Source: CAD feature listing. Evaluate the final solid. Frame: model axes, mm. Face numbers are marked on the shaded views. A direction names the side the tool comes from. Coordinates: 2 decimals unless noted, no trailing zeros. Order: outer loops, then holes, each group sorted by start corner. A loop starts at its lowest first (then second) coordinate and runs counter-clockwise, first axis right, second up. Notation, with made-up numbers: (63, -34) -> (115, -34) arc R22 cw to (115, -3) -> close; hole circle Ø5 at (79.5, -1). An arc over 180 degrees is marked (long way). Write item = value, one per line. Start each with the question number.
Item 1: Section query D-D (x = 23). Output: boundary loops of the cut face in (y, z), then the cut area to 3 significant figures.
Item 2: Set-up query: the marked faces 1 and 2. Return all of +Z, -Z, +X, -X, +Y, -Y with unobstructed straight access to the full face (end or side cutting, diameter ignored); none if empty.
Item 3: Section query C-C (y = 20). Output: boundary loops of the cut face in (x, z).
Item 4: Contact query for flat-ended pins moving along their axis: pin 1 (3 mm diameter, centred on y = 41.5, z = 18, fed in from -X); pin 2 (1.3 mm diameter, centred on y = 34.5, z = 10, fed in from +X); pin 3 (4 mm diameter, centred on y = 46.5, z = 17, fed in from +X); pin 4 (2 mm diameter, centred on x = -2.5, y = 30, fed in from +Z). Output: stop coordinate, or through.
Item 5: Ray query, line 1 along Z through (x, y) = (6.5, 31); line 2 along Y through (x, z) = (9, -0.5); line 3 along Y through (x, z) = (17, -0.5). Return the intervals inside material, ascending. Write a range as [from, to].
Item 6: Section query A-A (z = 18.5). Output: boundary loops of the cut face in (x, y), then the cut area to 3 significant figures.
Item 7: Section query B-B (x = 34). Output: boundary loops of the cut face in (y, z), then the cut area to 3 significant figures.
```python
from build123d import *

# Parameters (mm, degrees)
F0_W         = 25
F0_H         = 33
F1_DEPTH     = 25
F3_DEPTH     = 10
F5_DEPTH     = 81.7
F7_DEPTH     = 10
F9_DEPTH     = 92
F10_W        = 13
F10_H        = 13
F11_DEPTH    = 40
F12_R        = 1.9
F13_DEPTH    = 7
F15_DEPTH    = 2.5
F16_W        = 78.4268817365
F16_H        = 25
F17_DEPTH    = 2.5
F19_DEPTH    = 336
F21_DEPTH    = 25
F23_W        = 90.9570492804
F23_H        = 10.3441323154
F24_DEPTH    = 48.1
F26_DEPTH    = 199
F27_W        = 183.3121031523
F27_H        = 83.9067064226
F28_DEPTH    = 179
F29_T1_DEPTH = 32.3950995948
F29_T3_DEPTH = 10.395099863
F31_DEPTH    = 25
F32_R        = 1.9
F33_DEPTH    = 25


# Not quite as in the source:
# - a fillet or chamfer that OpenCascade refuses, or shapes differently, is made with other operations: its cross-section is extruded or revolved along the edge and cut away or added


with BuildPart() as f1:
    # F0 (on Top) → F1 (new body)
    with BuildSketch(Plane.XY):
        with Locations((12.5, 16.5)):
            Rectangle(F0_W, F0_H)
        Polygon((-25, 25.3567329635), (0, 0), (0, 33), align=None)
        with Locations((37.5, 16.5)):
            Rectangle(F0_W, F0_H)
        Polygon((25, 40.6432670365), (0, 33), (25, 33), align=None)
        Polygon((0, 101.4598330308), (0, 33), (25, 40.6432670365), (25, 101.4598330308), (25, 137), (0, 137), align=None)
        Polygon((25, 40.6432670365), (25, 33), (50, 33), (50, 48.2865340729), align=None)
        Polygon((-25, 131.6860859582), (0, 101.4598330308), (0, 137), align=None)
        Polygon((25, 137), (25, 101.4598330308), (50, 131.6860859582), (50, 147.6278280835), (25, 142.3139140418), align=None)
        Polygon((25, 142.3139140418), (0, 137), (25, 137), align=None)
        Polygon((0, 177), (0, 137), (25, 142.3139140418), (25, 177), align=None)
    extrude(amount=F1_DEPTH)

    # F2 (on face) → F3 (join)
    with BuildSketch(Plane(origin=(0, 0, 0), x_dir=(1, 0, 0), z_dir=(0, 0, -1))):
        Polygon((50, -131.6860859582), (25, -101.4598330308), (0, -101.4598330308), (-25, -131.6860859582), (50, -147.6278280835), align=None)
    extrude(amount=F3_DEPTH)

    # F4 (on face) → F5 (cut, symmetric)
    with BuildSketch(Plane.YZ.offset(25)):
        Polygon((101.4598330308, -21.1370438337), (147.6278330308, -10), (101.4598330308, 0), align=None)
    extrude(amount=F5_DEPTH, both=True, mode=Mode.SUBTRACT)

    # F6 (on face) → F7 (join)
    with BuildSketch(Plane(origin=(0, 0, 0), x_dir=(1, 0, 0), z_dir=(0, 0, -1))):
        Polygon((50, -48.2865340729), (50, 0), (0, 0), (-25, -25.3567329635), align=None)
    extrude(amount=F7_DEPTH)

    # F8 (on face) → F9 (cut)
    with BuildSketch(Plane.YZ.offset(50)):
        Polygon((48.2865340729, -10), (0, 0), (0, -39.534393698), (48.2865340729, -39.534393698), align=None)
    extrude(amount=-F9_DEPTH, mode=Mode.SUBTRACT)

    # F10 (on face) → F11 (cut)
    with BuildSketch(Plane(origin=(0, 177, 0), x_dir=(-1, 0, 0), z_dir=(0, 1, 0))):
        with Locations((-12.5, 12.5)):
            Rectangle(F10_W, F10_H)
    extrude(amount=-F11_DEPTH, mode=Mode.SUBTRACT)

    # F12 (on face) → F13 (cut)
    with BuildSketch(Plane(origin=(-27.8614600507, 131.0778638485, 0), x_dir=(-0.9781476007, -0.2079116908, 0), z_dir=(-0.2079116908, 0.9781476007, 0))):
        with Locations((-18.6253867704, 12.5)):
            Circle(F12_R)
        with BuildLine():
            ThreePointArc((-72.2009313853, 12.5), (-70.3009313853, 10.6), (-68.4009313853, 12.5))
            ThreePointArc((-68.4009313853, 12.5), (-70.3009313853, 14.4), (-72.2009313853, 12.5))
        make_face()
    extrude(amount=-F13_DEPTH, mode=Mode.SUBTRACT)

    # F15 (add): a face of the model
    f15_faces = [f1.faces().sort_by_distance(p)[0] for p in [
        (12.5, 36.8216335182, -0.8588233683),
    ]]
    extrude(f15_faces, amount=F15_DEPTH)

    # F16 (on face) → F17 (join)
    with BuildSketch(Plane(origin=(-9.9576121691, 32.5698818371, 0), x_dir=(-0.956304756, -0.2923717047, 0), z_dir=(-0.2923717047, 0.956304756, 0))):
        with Locations((-22.7194132119, 12.5)):
            Rectangle(F16_W, F16_H)
    extrude(amount=-F17_DEPTH)

    # F18 (on face) → F19 (cut)
    with BuildSketch(Plane(origin=(-9.9576121691, 32.5698818371, 0), x_dir=(-0.956304756, -0.2923717047, 0), z_dir=(-0.2923717047, 0.956304756, 0))):
        Polygon((16.4940276563, -15.7148446888), (16.4940276563, -3), (-61.9328540802, -3), (-74.3611752987, -3), (-74.3611752987, -15.7148446888), align=None)
    extrude(amount=-F19_DEPTH, mode=Mode.SUBTRACT)

    # F20 (on face) → F21 (cut)
    with BuildSketch(Plane.XY.offset(25)):
        Polygon((50, 48.2865340729), (-25, 25.3567329635), (-20.5921567976, -5.8456440456), (63.7660473585, -9.7692795098), align=None)
    extrude(amount=-F21_DEPTH, mode=Mode.SUBTRACT)

    # F23 (on offset) → F24 (cut)
    with BuildSketch(Plane(origin=(-6.30296586, 20.6160723875, 0), x_dir=(-0.956304756, -0.2923717047, 0), z_dir=(-0.2923717047, 0.956304756, 0))):
        with Locations((-20.5792468041, -2.5766163599)):
            Rectangle(F23_W, F23_H)
    extrude(amount=-F24_DEPTH, mode=Mode.SUBTRACT)

    # F25 (on face) → F26 (cut)
    with BuildSketch(Plane(origin=(0, 177, 0), x_dir=(-1, 0, 0), z_dir=(0, 1, 0))):
        Polygon((0.3, 25), (0, 25), (-25, 25), (-25.3, 25), (-25.3, 0), (-25, 0), (0, 0), (0.3, 0), align=None)
    extrude(amount=-F26_DEPTH, mode=Mode.SUBTRACT)

    # F27 (on face) → F28 (cut)
    with BuildSketch(Plane(origin=(-9.9576121691, 32.5698818371, 0), x_dir=(-0.956304756, -0.2923717047, 0), z_dir=(-0.2923717047, 0.956304756, 0))):
        with Locations((-51.5790507197, 11.8016507477)):
            Rectangle(F27_W, F27_H)
    extrude(amount=F28_DEPTH, mode=Mode.SUBTRACT)

    # F29: fillet of radius 3 on 1 edges, made by hand

    # F29_s2 → F29_t1 (cut)
    with BuildSketch(Plane.XY.offset(1.341e-07)):
        with BuildLine():
            ThreePointArc((-25, 25.3567329635), (-24.5468104619, 27.3684218455), (-22.9021416452, 28.6123420192))
            Line((-22.9021416452, 28.6123420192), (-25.7309292618, 27.7474948534))
            Line((-25.7309292618, 27.7474948534), (-25, 25.3567329635))
        make_face()
    extrude(amount=F29_T1_DEPTH, mode=Mode.SUBTRACT)

    # F29_s4 → F29_t3 (cut)
    with BuildSketch(Plane.XY.offset(-10.3950997289)):
        with BuildLine():
            ThreePointArc((-25, 25.3567329635), (-24.5468104619, 27.3684218455), (-22.9021416452, 28.6123420192))
            Line((-22.9021416452, 28.6123420192), (-25.7309292618, 27.7474948534))
            Line((-25.7309292618, 27.7474948534), (-25, 25.3567329635))
        make_face()
    extrude(amount=F29_T3_DEPTH, mode=Mode.SUBTRACT)

    # F30 (on face) → F31 (cut)
    with BuildSketch(Plane(origin=(-9.2266829073, 30.1791199472, 0), x_dir=(0.956304756, 0.2923717047, 0), z_dir=(0.2923717047, -0.956304756, 0))):
        with BuildLine():
            ThreePointArc((-3.3940276563, 12.5), (-1.4940276563, 10.6), (0.4059723437, 12.5))
            ThreePointArc((0.4059723437, 12.5), (-1.4940276563, 14.4), (-3.3940276563, 12.5))
        make_face()
    extrude(amount=-F31_DEPTH, mode=Mode.SUBTRACT)

    # F32 (on face) → F33 (cut)
    with BuildSketch(Plane(origin=(-9.2266829073, 30.1791199472, 0), x_dir=(0.956304756, 0.2923717047, 0), z_dir=(0.2923717047, -0.956304756, 0))):
        with Locations((51.9328540802, 12.5)):
            Circle(F32_R)
    extrude(amount=-F33_DEPTH, mode=Mode.SUBTRACT)


solid = f1.part
```
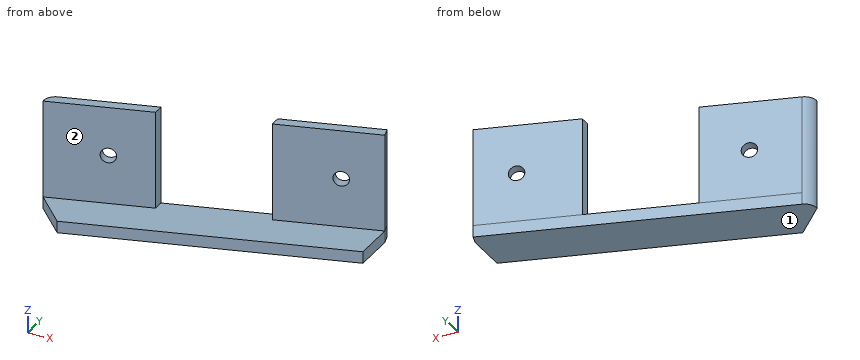
Computed:
q1.outline = (29.57, -3) -> (42.65, -3) -> (42.65, 0) -> (29.57, 0) -> close
q1.area = 39.2 mm^2
q2.face_1 = -Z, +X, -X, +Y, -Y
q2.face_2 = +Z, +X, -Y
q3.outline = (-19.72, -3) -> (-8.32, -3) -> (-8.32, 0) -> (-19.72, 0) -> close
q4.pin_1 = 25.3
q4.pin_2 = -0.3
q4.pin_3 = 50
q4.pin_4 = 0
q5.line_1 = [-3, 0]
q5.line_2 = [25.29, 38.37]
q5.line_3 = [27.74, 40.81]
q6.outline = (-25, 25.36) -> (-0.3, 32.91) -> (-0.3, 35.52) -> (-22.9, 28.61) arc R3 ccw to start; (25.3, 40.73) -> (50, 48.29) -> (49.27, 50.68) -> (25.3, 43.35) -> close
q6.area = 127 mm^2
q7.outline = (32.94, -3) -> (46.01, -3) -> (46.01, 25) -> (43.39, 25) -> (43.39, 0) -> (32.94, 0) -> close
q7.area = 105 mm^2
